Geometry: final body of the model. Coordinates: model frame, mm. A direction names the side the tool comes from. Give positions to 0.01 mm unless a question says otherwise; leave off trailing zeros. Order: outer loops, then holes, each group sorted by start corner. A loop starts at its lowest first (then second) coordinate and runs counter-clockwise, first axis right, second up. Notation, with made-up numbers: (87.5, -27) - (122.5, -27) arc R13 ccw to (122.5, -12) - close; hole circle Ø10 at (18, -39). An arc over 180 degrees is marked (long way). Put each result on its own line as item: value. Start each with the question number.
1. Set-up query: faces 5 (the flat face through (47.75, 0, 7)), 6 (the flat face through (-1, 3, 9)), 7 (the flat face through (1, 5, 4)), 8 (the flat face through (-54, -4, 4)). Return all of +Z, -Z, +X, -X, +Y, -Y with unobstructed straight access to the full face (end or side cutting, diameter ignored); none if empty.
2. Mould query, pull axis X, two halves, no side actions, for faces 1 (the cylindrical face through (51.022, 7.966, 4.437)), 2 (the cylindrical face through (56.9, 11.93, 4.44)), 3 (the cylindrical face through (-56.93, -11.9, 4.56)), 4 (the flat face through (-1, 0, 0)). Classes: pulls with the +X half, pulls with the -X half, needs draft (parallel to the pull), parting line crosses it, or undercut.
3. Ray query, line 1 along Y through (x, z) = (52.5, 4.5); line 2 along X through (y, z) = (-7.5, 4.5); line 3 along Y through (x, z) = (-52.5, 6.75). Return the intervals inside material, ascending. Write a range as from..to.
4. Section A-A on x = -52.5. Return the cut outline in (y, z).
5. Section B-B on y = -7.5. Return the cut outline in (x, z), plus the area to 3 significant figures.
6. Section D-D on x = 20. Return the cut outline in (y, z).
7. Section C-C on z = 8. Return the cut outline in (x, y).
from build123d import *

# Parameters (mm, degrees)
SKETCH_W              = 115
SKETCH_H              = 25
PAD_DEPTH             = 3
PAD001_DEPTH          = 3
SKETCH002_W           = 115
SKETCH002_H           = 25
SKETCH002_W_2         = 95.5
SKETCH002_H_2         = 3
PAD002_DEPTH          = 3
SKETCH003_R           = 1.55
POCKET_DEPTH          = 245.060315
POLARPATTERN_COUNT    = 2
POLARPATTERN001_COUNT = 2
POLARPATTERN002_COUNT = 2
FILLET_R              = 2


with BuildPart() as part:
    # Sketch → Pad (new body)
    with BuildSketch(Plane.XY):
        Rectangle(SKETCH_W, SKETCH_H)
    extrude(amount=PAD_DEPTH)

    # Sketch001 (on Face6 of Pad) → Pad001 (join)
    with BuildSketch(Plane.XY.offset(3)):
        Polygon((-57.5, 12.5), (57.5, 12.5), (57.5, 4), (50, 4), (50, 5), (-50, 5), (-50, 4), (-57.5, 4), align=None)
        Polygon((-57.5, -12.5), (57.5, -12.5), (57.5, -4), (50, -4), (50, -5), (-50, -5), (-50, -4), (-57.5, -4), align=None)
    extrude(amount=PAD001_DEPTH)

    # Sketch002 (on Face12 of Pad001) → Pad002 (join)
    with BuildSketch(Plane.XY.offset(6)):
        Rectangle(SKETCH002_W, SKETCH002_H)
        Rectangle(SKETCH002_W_2, SKETCH002_H_2, mode=Mode.SUBTRACT)
    extrude(amount=PAD002_DEPTH)

    # Sketch003 (on Face26 of Pad002) → Pocket (cut, through all)
    with BuildSketch(Plane.XY.offset(9)):
        with Locations((-52.5, 7.5)):
            Circle(SKETCH003_R)
    pocket = extrude(amount=-POCKET_DEPTH, mode=Mode.SUBTRACT)

    # PolarPattern: Pocket ×2 about axis
    polarpattern_axis = Axis((0, 0, 0), (0, 1, 0))
    for i in range(1, POLARPATTERN_COUNT):
        add(pocket.rotate(polarpattern_axis, i * 360 / POLARPATTERN_COUNT), mode=Mode.SUBTRACT)

    # PolarPattern001: Pocket ×2 about axis
    polarpattern001_axis = Axis((0, 0, 0), (1, 0, 0))
    for i in range(1, POLARPATTERN001_COUNT):
        add(pocket.rotate(polarpattern001_axis, i * 360 / POLARPATTERN001_COUNT), mode=Mode.SUBTRACT)

    # PolarPattern002: Pocket ×2 about axis
    polarpattern002_axis = Axis((0, 0, 9), (0, 0, 1))
    for i in range(1, POLARPATTERN002_COUNT):
        add(pocket.rotate(polarpattern002_axis, i * 360 / POLARPATTERN002_COUNT), mode=Mode.SUBTRACT)

    # Fillet
    fillet_edges = [part.edges().sort_by_distance(p)[0] for p in [
        (57.5, 12.5, 7.5),
        (57.5, 12.5, 4.5),
        (57.5, 12.5, 1.5),
        (57.5, -12.5, 7.5),
        (-57.5, 12.5, 7.5),
        (-57.5, -12.5, 7.5),
    ]]
    fillet(fillet_edges, radius=FILLET_R)


solid = part.part
Resolved:
1. face 5: +Z
1. face 6: +Z, +X, -X, +Y, -Y
1. face 7: none
1. face 8: +X, -X
2. face 1: undercut
2. face 2: pulls with the +X half
2. face 3: pulls with the -X half
2. face 4: needs draft
3. line 1: -12.5..-9.05, -5.95..-4, 4..5.95, 9.05..12.5
3. line 2: -57.5..-54.05, -50.95..50.95, 54.05..57.5
3. line 3: -12.5..-9.05, -5.95..5.95, 9.05..12.5
4. outline: (-12.5, 0) - (-9.05, 0) - (-9.05, 9) - (-12.5, 9) - close; (-5.95, 0) - (5.95, 0) - (5.95, 9) - (-5.95, 9) - close; (9.05, 0) - (12.5, 0) - (12.5, 9) - (9.05, 9) - close; hole (-4, 3) - (4, 3) - (4, 6) - (-4, 6) - close
5. outline: (-57.5, 0) - (-54.05, 0) - (-54.05, 9) - (-57.5, 9) - close; (-50.95, 0) - (50.95, 0) - (50.95, 9) - (-50.95, 9) - close; (54.05, 0) - (57.5, 0) - (57.5, 9) - (54.05, 9) - close
5. area: 979 mm^2
6. outline: (-12.5, 0) - (12.5, 0) - (12.5, 9) - (1.5, 9) - (1.5, 6) - (5, 6) - (5, 3) - (-5, 3) - (-5, 6) - (-1.5, 6) - (-1.5, 9) - (-12.5, 9) - close
7. outline: (-57.5, -10.5) arc R2 ccw to (-55.5, -12.5) - (55.5, -12.5) arc R2 ccw to (57.5, -10.5) - (57.5, 10.5) arc R2 ccw to (55.5, 12.5) - (-55.5, 12.5) arc R2 ccw to (-57.5, 10.5) - close; hole circle Ø3.1 at (-52.5, -7.5); hole circle Ø3.1 at (-52.5, 7.5); hole (-47.75, -1.5) - (47.75, -1.5) - (47.75, 1.5) - (-47.75, 1.5) - close; hole circle Ø3.1 at (52.5, -7.5); hole circle Ø3.1 at (52.5, 7.5)
